Source: three-view drawing plus pictorial views. Frame: mm from the lowest corner of the part. A direction names the side the tool comes from. Coordinates: 2 decimals unless noted, no trailing zeros. Order: outer loops, then holes, each group sorted by start corner. A loop starts at its lowest first (then second) coordinate and runs counter-clockwise, first axis right, second up. Notation, with made-up numbers: (62, 31.5) -> (111, 31.5) arc R34 ccw to (111, 62.5) -> close; hole circle Ø4 at (24, 85). An arc over 180 degrees is marked (long way). Use one line per item in the form item = value. Start each with the question number.
1) Pin query (flat end, axial travel): pin 1 (3 mm diameter, centred on x = 71, y = 183.5, fed in from +Z); pin 2 (2 mm diameter, centred on x = 57, z = 29, fed in from +Y); pin 3 (10 mm diameter, centred on y = 158.5, z = 66.5, fed in from +X). Return the tip coordinate at first contact, or that it passes through.
2) Access query for the marked faces 4 and 5. Directions: +Z, -Z, +X, -X, +Y, -Y. A direction counts if a zero-diameter tool reaches every point of the face in a straight line with its end or side. Return the directions, or none.
3) Section query C-C on z = 16. Output: boundary loops of the cut face in (x, y).
4) Ray query, line 1 along X through (y, z) = (110, 42); line 2 along Y through (x, z) = (114, 53). Return the intervals inside material, ascending.
5) Draft query along Y for the marked faces 1, 2 and 3. Return one class per face: pulls with the +Y half, pulls with the -Y half, needs draft (parallel to the pull), parting line crosses it, or undercut.
6) Section query A-A on x = 110. Output: boundary loops of the cut face in (y, z), then the cut area to 3 significant figures.
7) Section query D-D on x = 177. Output: boundary loops of the cut face in (y, z), then the cut area to 3 significant figures.
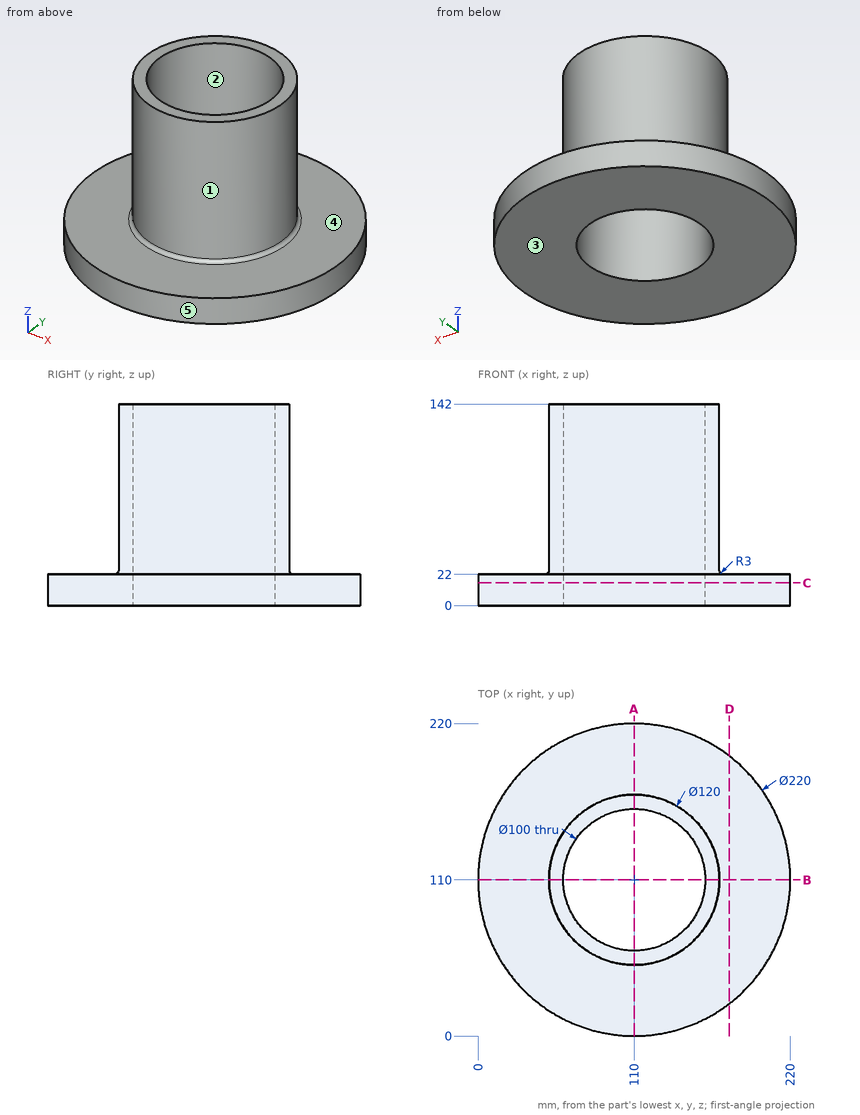
Answers below:
q1.pin_1 = 22
q1.pin_2 = 139.93
q1.pin_3 = 151.32
q2.face_4 = +Z
q2.face_5 = +Z, -Z
q3.outline = circle Ø220 at (110, 110); hole circle Ø100 at (110, 110)
q4.line_1 = 50 to 60, 160 to 170
q4.line_2 = 50.13 to 60.16, 159.84 to 169.87
q5.face_1 = parting line crosses it
q5.face_2 = undercut
q5.face_3 = needs draft
q6.outline = (0, 0) -> (60, 0) -> (60, 142) -> (50, 142) -> (50, 25) arc R3 cw to (47, 22) -> (0, 22) -> close; (160, 0) -> (220, 0) -> (220, 22) -> (173, 22) arc R3 cw to (170, 25) -> (170, 142) -> (160, 142) -> close
q6.area = 5,040 mm^2
q7.outline = (22.76, 0) -> (197.24, 0) -> (197.24, 22) -> (22.76, 22) -> close
q7.area = 3,840 mm^2
